Here's how the part is built. I have some questions about the finished solid (model axes, mm). Face numbers are marked on the shaded views. Round coordinates to 2 decimals unless told otherwise and drop trailing zeros. Order: outer loops, then holes, each group sorted by start corner. A loop starts at its lowest first (then second) coordinate and runs counter-clockwise, first axis right, second up. Notation, with made-up numbers: (78.25, -32) -> (116.25, -32) arc R21 ccw to (116.25, -2) -> close; hole circle Ø7 at (29, 7). An arc over 180 degrees is marked (long way). One line per item, written item: value.
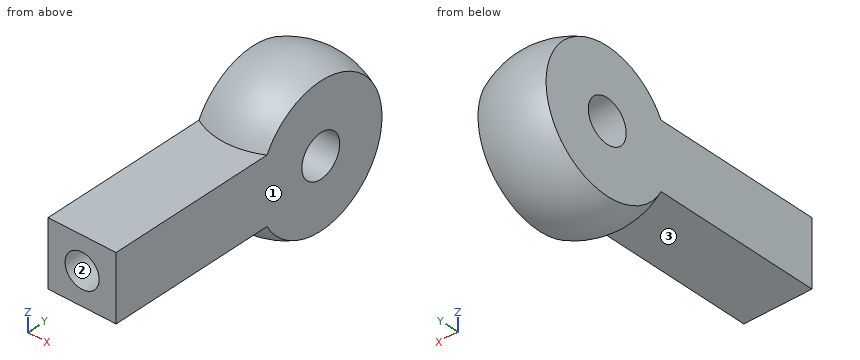
```python
from build123d import *

# Parameters (mm, degrees)
CUT_EXTRUDE_START        = -9
CUT_EXTRUDE_1_OUTLINE_W  = 6
CUT_EXTRUDE_1_OUTLINE_H  = 20
CUT_EXTRUDE_1_DEPTH      = 18
CUT_EXTRUDE_2_DEPTH      = 19.193405399
CUT_EXTRUDE_2_DEPTH_BACK = 19.193405399
SKETCH_3_R               = 2.5
SKETCH_4_W               = 7.669123848
SKETCH_4_H               = 20.676781993
EXTRUDE_1_DEPTH          = 8
SKETCH_5_R               = 2
CUT_EXTRUDE_3_DEPTH      = 15


with BuildPart() as part:
    # 草图1 → 旋转1 (revolve)
    with BuildSketch(Plane(origin=(0, 0, 0), x_dir=(0, 0, -1), z_dir=(1, 0, 0))):
        with BuildLine():
            Line((0, 9), (0, -9))
            ThreePointArc((0, -9), (-9, 0), (0, 9))
        make_face()
    revolve(axis=Axis((0, 9, 0), (0, -1, 0)))

    # 切除-拉伸1: read off the stored shape, not the designer's step
    # 切除-拉伸1 outline → 切除-拉伸1 (cut)
    with BuildSketch(Plane.XY.offset(CUT_EXTRUDE_START)):
        with Locations((-7, 0)):
            Rectangle(CUT_EXTRUDE_1_OUTLINE_W, CUT_EXTRUDE_1_OUTLINE_H)
        with Locations((7, 0)):
            Rectangle(CUT_EXTRUDE_1_OUTLINE_W, CUT_EXTRUDE_1_OUTLINE_H)
    extrude(amount=CUT_EXTRUDE_1_DEPTH, mode=Mode.SUBTRACT)

    # 草图3 → 切除-拉伸2 (cut, two sides: drawn at the far end of the back side and taken through both)
    with BuildSketch(Plane(origin=(4, 0, 0), x_dir=(0, 0, -1), z_dir=(1, 0, 0)).offset(-CUT_EXTRUDE_2_DEPTH_BACK)):
        Circle(SKETCH_3_R)
    extrude(amount=CUT_EXTRUDE_2_DEPTH + CUT_EXTRUDE_2_DEPTH_BACK, mode=Mode.SUBTRACT)

    # 草图4 → 凸台-拉伸1 (add)
    with BuildSketch(Plane(origin=(4, 0, 0), x_dir=(0, 0, -1), z_dir=(1, 0, 0))):
        with Locations((0, -16.661609004)):
            Rectangle(SKETCH_4_W, SKETCH_4_H)
    extrude(amount=-EXTRUDE_1_DEPTH)

    # 草图5 → 切除-拉伸3 (cut)
    with BuildSketch(Plane.XZ.offset(27)):
        with Locations(Location((0, 0, 0), (0, 0, 270))):
            Circle(SKETCH_5_R)
    extrude(amount=-CUT_EXTRUDE_3_DEPTH, mode=Mode.SUBTRACT)


solid = part.part
```
Q1. I need wall thicknesses on line 1 along X through (y, z) = (-21, 0); line 2 along Y through (x, z) = (-1, 0); line 3 along Y through (x, z) = (-1.5, 8). Which ranges of each line are inside material? Lowest first, please.
Answers:
line 1: -4 to -2, 2 to 4
line 2: -12 to -2.5, 2.5 to 8.94
line 3: -3.84 to 3.84
Q2. If we mould it in two halves opening along Z, with no side actions, what happens to the marked faces 1, 2 and 3? For each: pulls with the +Z half, pulls with the -Z half, needs draft (parallel to the pull), parting line crosses it, or undercut.
Answers:
face 1: needs draft
face 2: undercut
face 3: pulls with the -Z half
Q3. For P1, Ø1, axis at x = 0.5, y = -23, coming from the -Z side; P2, Ø2.5, axis at x = -0.5, y = -19, coming from the +Z side; P3, Ø3, axis at y = 0, z = 0, coming from the +X side, each with a flat end and sliding along its axis, tell me the tip position at first contact or that it passes through.
Answers:
P1: z = -3.83
P2: z = 3.83
P3: through
Q4. I want a section at B-B on z = 0. Write out the boundary of the cut face in (x, y), then the cut area to 3 significant figures.
Answers:
outline: (-4, -27) -> (-2, -27) -> (-2, -12) -> (2, -12) -> (2, -27) -> (4, -27) -> (4, -2.5) -> (-4, -2.5) -> close; (-4, 2.5) -> (4, 2.5) -> (4, 8.06) arc R9 ccw to (-4, 8.06) -> close
area: 186 mm2
Q5. I want a section at D-D on y = -13.5. Write out the boundary of the cut face in (x, z).
Answers:
outline: (-4, -3.83) -> (4, -3.83) -> (4, 3.83) -> (-4, 3.83) -> close; hole circle Ø4 at (0, 0)
Q6. I want a section at C-C on x = 1.25. Write out the boundary of the cut face in (y, z).
Answers:
outline: (-27, -3.83) -> (-8.05, -3.83) arc R8.91 ccw (long way) to (-8.05, 3.83) -> (-27, 3.83) -> (-27, 1.56) -> (-12, 1.56) -> (-12, -1.56) -> (-27, -1.56) -> close; hole circle Ø5 at (0, 0)
Q7. I want a section at A-A on y = 0. Write out the boundary of the cut face in (x, z), then the cut area to 3 significant figures.
Answers:
outline: (-4, -8.06) arc R9 ccw to (4, -8.06) -> (4, -2.5) -> (-4, -2.5) -> close; (-4, 2.5) -> (4, 2.5) -> (4, 8.06) arc R9 ccw to (-4, 8.06) -> close
area: 99.1 mm2
